Check sheet for the modelled part. Datum: model origin and axes. Units: mm. Face numbers are marked on the shaded views. Coordinates: 2 decimals unless noted, no trailing zeros. Loops run counter-clockwise (first coordinate to the right, second up) from the corner with the lowest first, then second, coordinate; pieces in that order, holes last. Notation, with made-up numbers: (-18.5, 82.25) - (-10.5, 82.25) arc R26 cw to (-10.5, 102.25) - close; hole circle Ø5 at (-39.5, 78). An arc over 180 degrees is marked (long way). Use a Markdown table: item, result. Add a question column.
1) Sectioned sample at A-A, the plane y = 17. Enter the section's corners in (x, z), then the cut area to 3 significant figures.
2) Thickness scan on line 1 (X direction, y = 41, z = -7.5); line 2 (Z direction, x = -70, y = 17); line 3 (X direction, y = 53, z = 1.25). Record the ranges inside material, lowest first.
3) Go/stop test with flat-tipped pins: P1, Ø3, axis at x = 70, z = -7.5, coming from the -Y side; P2, Ø1, axis at x = 1, z = -10.5, coming from the +Y side; P3, Ø4, axis at x = 19.5, y = 62, coming from the -Z side. Record where each tip stops, or that it passes through.
4) Sectioned sample at C-C, the plane z = -7.5. Enter the section's corners in (x, y).
5) Sectioned sample at D-D, the plane z = -0.5. Enter the section's corners in (x, y).
6) Draft check along Y on the marked faces 1, 2 and 3. Enter one of: pulls with the +Y half, pulls with the -Y half, needs draft (parallel to the pull), parting line crosses it, or undercut.
7) Sectioned sample at B-B, the plane x = -70. Enter the section's corners in (y, z), then the cut area to 3 significant figures.
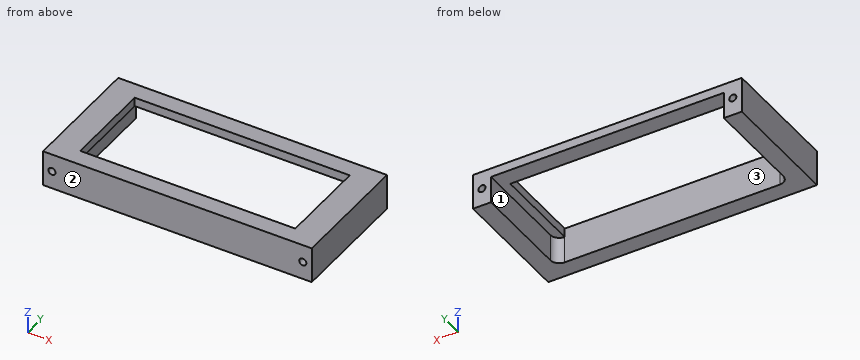
from build123d import *

# Parameters (mm, degrees)
SKETCH1_W                = 130
SKETCH1_H                = 5
BOSS_EXTRUDE1_DEPTH      = 69
SKETCH2_W                = 120
SKETCH2_H                = 50
CUT_EXTRUDE1_DEPTH       = 65
BOSS_EXTRUDE3_DEPTH      = 15
BOSS_EXTRUDE3_DEPTH_BACK = 5
SKETCH4_R                = 2
CUT_EXTRUDE2_DEPTH       = 70
FILLET1_R                = 5


with BuildPart() as part:
    # Sketch1 → Boss-Extrude1 (new body)
    with BuildSketch(Plane(origin=(0, 0, 0), x_dir=(1, 0, 0), z_dir=(0, 1, 0))):
        Rectangle(SKETCH1_W, SKETCH1_H)
    extrude(amount=BOSS_EXTRUDE1_DEPTH)

    # Sketch2 → Cut-Extrude1 (cut)
    with BuildSketch(Plane.XY.offset(2.5)):
        with Locations((0, 34.5)):
            Rectangle(SKETCH2_W, SKETCH2_H)
    extrude(amount=-CUT_EXTRUDE1_DEPTH, mode=Mode.SUBTRACT)

    # Sketch3 → Boss-Extrude3 (add, two sides)
    with BuildSketch(Plane(origin=(0, 0, -2.5), x_dir=(-1, 0, 0), z_dir=(0, 0, -1))) as boss_extrude3_sk:
        Polygon((75, 0), (-75, 0), (-75, 69), (-65, 69), (-65, 9.5), (65, 9.5), (65, 69), (75, 69), align=None)
    extrude(amount=BOSS_EXTRUDE3_DEPTH)
    extrude(boss_extrude3_sk.sketch, amount=-BOSS_EXTRUDE3_DEPTH_BACK)

    # Sketch4 → Cut-Extrude2 (cut, through all)
    with BuildSketch(Plane(origin=(0, 69, 0), x_dir=(1, 0, 0), z_dir=(0, 1, 0))):
        with Locations((-70, 7.5)):
            Circle(SKETCH4_R)
        with Locations((70, 7.5)):
            Circle(SKETCH4_R)
    extrude(amount=-CUT_EXTRUDE2_DEPTH, mode=Mode.SUBTRACT)

    # Fillet1
    fillet1_edges = [part.edges().sort_by_distance(p)[0] for p in [
        (65, 9.5, -10),
        (-65, 9.5, -10),
    ]]
    fillet(fillet1_edges, radius=FILLET1_R)


solid = part.part
Solved:
| question | item | result |
|---|---|---|
| 1 | outline | (-75, -17.5) - (-65, -17.5) - (-65, -2.5) - (-60, -2.5) - (-60, 2.5) - (-75, 2.5) - close; (60, -2.5) - (65, -2.5) - (65, -17.5) - (75, -17.5) - (75, 2.5) - (60, 2.5) - close; hole circle Ø4 at (-70, -7.5); hole circle Ø4 at (70, -7.5) |
| 1 | area | 425 mm2 |
| 2 | line 1 | x = -75 to -72, -68 to -65, 65 to 68, 72 to 75 |
| 2 | line 2 | z = -17.5 to -9.5, -5.5 to 2.5 |
| 2 | line 3 | x = -75 to -60, 60 to 75 |
| 3 | P1 | passes through |
| 3 | P2 | stops at y = 9.5 |
| 3 | P3 | stops at z = -2.5 |
| 4 | outline | (-75, 0) - (-72, 0) - (-72, 69) - (-75, 69) - close; (-68, 0) - (68, 0) - (68, 69) - (65, 69) - (65, 14.5) arc R5 cw to (60, 9.5) - (-60, 9.5) arc R5 cw to (-65, 14.5) - (-65, 69) - (-68, 69) - close; (72, 0) - (75, 0) - (75, 69) - (72, 69) - close |
| 5 | outline | (-75, 0) - (75, 0) - (75, 69) - (-75, 69) - close; hole (-60, 9.5) - (60, 9.5) - (60, 59.5) - (-60, 59.5) - close |
| 6 | face 1 | needs draft |
| 6 | face 2 | pulls with the -Y half |
| 6 | face 3 | undercut |
| 7 | outline | (0, -17.5) - (69, -17.5) - (69, -9.5) - (0, -9.5) - close; (0, -5.5) - (69, -5.5) - (69, 2.5) - (0, 2.5) - close |
| 7 | area | 1,100 mm2 |
